Build history of the part. All positions in model axes, mm. A direction names the side the tool comes from. Coordinates: 2 decimals unless noted, no trailing zeros. Loops run counter-clockwise (first coordinate to the right, second up) from the corner with the lowest first, then second, coordinate; pieces in that order, holes last.
(1) Tool access for faces 1 (the face through (56, 12.6, 17)), 2 (the face through (9.3, 18, 17)), 3 (the face through (35, 10, 5)): list every direction of +Z, -Z, +X, -X, +Y, -Y with a clear straight run to the whole face (end or side of a thin tool).
(2) Slice it at B-B (y = 22.5). Give the cut face in (x, z), and give its area (3 significant figures).
(3) Slice it at D-D (y = 7). Give the cut face in (x, z), and give its area (3 significant figures).
(4) Two-plate mould, pull along X, no slides. Class faces 4 (the face through (53.6, 18, 17)), 5 (the face through (58.6, 18, 15)), 6 (the face through (41.9, 24, 4.8)), 7 (the face through (30.7, 18, 17)): pulls with the +X half, pulls with the -X half, needs draft (parallel to the pull), parting line crosses it, or undercut.
(5) Flat gauge pins, fed straight in: P1, Ø4, axis at y = 18.3, z = 19, coming from the +X side; P2, Ø1.5, axis at x = 12, z = 20, coming from the -Y side; P3, Ø1, axis at x = 46, y = 3.5, coming from the +Z side; P4, Ø6.5, axis at x = 29, y = 7, coming from the -Z side. Where does each tip first touch, or does it go through?
(6) Wall check: L1, parallel to Z at x = 27.75, y = 18.3; L2, parallel to X at y = 18, z = 12.5; L3, parallel to Y at x = 60, z = 2.85. Give the ranges that are in metal, low to high.
(7) Slice it at C-C (z = 28). Give the cut face in (x, y), and give its area (3 significant figures).
(8) Slice it at A-A (x = 29). Give the cut face in (y, z).
from build123d import *

# Parameters (mm, degrees)
SKETCH_W        = 70
SKETCH_H        = 24
SKETCH_R        = 2
PAD_DEPTH       = 5
SKETCH001_W     = 11.4
SKETCH001_H     = 11.4
POCKET_DEPTH    = 5.001
SKETCH002_W     = 5
SKETCH002_H     = 11.4
PAD001_DEPTH    = 25
SKETCH003_R     = 1.5
POCKET001_DEPTH = 58.601


with BuildPart() as part:
    # Sketch → Pad (new body)
    with BuildSketch(Plane.XY):
        with Locations((35, 12)):
            Rectangle(SKETCH_W, SKETCH_H)
        with Locations((60, 7)):
            Circle(SKETCH_R, mode=Mode.SUBTRACT)
        with Locations((29, 7)):
            Circle(SKETCH_R, mode=Mode.SUBTRACT)
    extrude(amount=PAD_DEPTH)

    # Sketch001 → Pocket (cut, through all)
    with BuildSketch(Plane.XY.offset(5)):
        with Locations((64.3, 18.3)):
            Rectangle(SKETCH001_W, SKETCH001_H)
        with Locations((20, 18.3)):
            Rectangle(SKETCH001_W, SKETCH001_H)
    extrude(amount=-POCKET_DEPTH, mode=Mode.SUBTRACT)

    # Sketch002 → Pad001 (new body)
    with BuildSketch(Plane.XY.offset(5)):
        with Locations((11.8, 18.3)):
            Rectangle(SKETCH002_W, SKETCH002_H)
        with Locations((28.2, 18.3)):
            Rectangle(SKETCH002_W, SKETCH002_H)
        with Locations((56.1, 18.3)):
            Rectangle(SKETCH002_W, SKETCH002_H)
    extrude(amount=PAD001_DEPTH)

    # Sketch003 → Pocket001 (cut, through all)
    with BuildSketch(Plane.YZ.offset(58.6)):
        with Locations((18.3, 19)):
            Circle(SKETCH003_R)
        with Locations((18.3, 11)):
            Circle(SKETCH003_R)
    extrude(amount=-POCKET001_DEPTH, mode=Mode.SUBTRACT)


solid = part.part
Response values:
1. face 1: +Z, +X, -X, -Y
1. face 2: +Z, -X, +Y, -Y
1. face 3: +Z, -Y
2. outline: (0, 0) - (14.3, 0) - (14.3, 30) - (9.3, 30) - (9.3, 5) - (0, 5) - close; (25.7, 0) - (58.6, 0) - (58.6, 30) - (53.6, 30) - (53.6, 5) - (30.7, 5) - (30.7, 30) - (25.7, 30) - close
2. area: 611 mm2
3. outline: (0, 0) - (27, 0) - (27, 5) - (0, 5) - close; (31, 0) - (58, 0) - (58, 5) - (31, 5) - close; (62, 0) - (70, 0) - (70, 5) - (62, 5) - close
3. area: 310 mm2
4. face 4: undercut
4. face 5: pulls with the +X half
4. face 6: needs draft
4. face 7: undercut
5. P1: stops at x = 58.6
5. P2: stops at y = 12.6
5. P3: stops at z = 5
5. P4: stops at z = 0
6. L1: z = 0 to 9.5, 12.5 to 17.5, 20.5 to 30
6. L2: x = 9.3 to 14.3, 25.7 to 30.7, 53.6 to 58.6
6. L3: y = 0 to 5, 9 to 12.6
7. outline: (9.3, 12.6) - (14.3, 12.6) - (14.3, 24) - (9.3, 24) - close; (25.7, 12.6) - (30.7, 12.6) - (30.7, 24) - (25.7, 24) - close; (53.6, 12.6) - (58.6, 12.6) - (58.6, 24) - (53.6, 24) - close
7. area: 171 mm2
8. outline: (0, 0) - (5, 0) - (5, 5) - (0, 5) - close; (9, 0) - (24, 0) - (24, 30) - (12.6, 30) - (12.6, 5) - (9, 5) - close; hole circle Ø3 at (18.3, 11); hole circle Ø3 at (18.3, 19)
